Build history of the part. All positions in model axes, mm. A direction names the side the tool comes from. Round coordinates to 2 decimals unless told otherwise and drop trailing zeros. Write each loop counter-clockwise with the first axis right and the second up, starting at its lowest first coordinate (ties: lowest second). Pieces come first, ordered by that corner, then holes.
Item 1: Drop flat-ended pins along their axis: pin 1 Ø3 at (x, z) = (29.5, -20.5) entering from -Y; pin 2 Ø8 at (y, z) = (-28.99, -28.99) entering from +X (3 decimals); pin 3 Ø5 at (x, y) = (15, -27.5) entering from -Z; pin 4 Ø2.5 at (x, y) = (34.5, 27) entering from +Z. Give the stop position or say it passes through.
Item 2: Band-saw the part on A-A, the plane x = 35. Write the cut outline in (y, z).
Item 3: Band-saw the part on C-C, the plane x = 27.5. Write the cut outline in (y, z).
Item 4: Band-saw the part on B-B, the plane x = 6. Write the cut outline in (y, z), then the cut area to 3 significant figures.
Item 5: Wall check: probe 1 along Z at (x, y) = (1.95, 0); probe 2 along Z at (x, y) = (7, 0); probe 3 along Z at (x, y) = (11, -33). Give the ranges that are in metal, low to high.
Item 6: Mould opens along Z. For faces 1 (the flat face through (34, -26, 4)), 2 (the flat face through (31, 0, -26)), 3 (the cylindrical face through (6.577, 49.787, -11.056)) say: +Z half, -Z half, draft (parallel to the pull), parting line (faces both ways), or undercut.
Item 7: 3-axis set-ups, long thin cutter, end or side, ignore diameter. For faces 4 (the conical face through (11.19, 6.17, 11.87)), 5 (the flat face through (22, 21, 21)), 6 (the flat face through (1, 12, 6)), 7 (the flat face through (35, -4, -26)), 8 (the flat face through (34, 26, 4)): which of +Z, -Z, +X, -X, +Y, -Y reach the whole face in a straight line?
Autodesk Inventor part; units mm, degrees
ref_plane "YZ Plane" through (0, 0, 0) normal (1, 0, 0) x (0, 1, 0)
ref_plane "XZ Plane" through (0, 0, 0) normal (0, 1, 0) x (-1, 0, 0)
ref_plane "XY Plane" through (0, 0, 0) normal (0, 0, 1) x (1, 0, 0)
sketch "草图1" plane through (0, 0, 0) normal (0, 1, 0) x (-1, 0, 0)
  line L0 (0, 51) -> (-12, 51)
  line L1 (-12, 51) -> (-12, 29)
  line L2 (-12, 29) -> (-14.5, 29)
  line L3 (-14.5, 29) -> (-14.5, 31)
  line L4 (-14.5, 31) -> (-22, 31)
  line L5 (-22, 31) -> (-22, 29)
  line L6 (-22, 29) -> (-38, 29)
  line L7 (-38, 29) -> (-38, 0)
  line L8 (-38, 0) -> (0, 0)
  line L9 (0, 0) -> (0, 51)
  line L10 (0, 29) -> (-1, 28)
  line L11 (-1, 28) -> (-1, 0)
  line L12 (-38, 25) -> (-15, 22.6998)
  line L13 (-15, 22.6998) -> (-15, 0)
  line L14 (7.6, 0) -> (-45.6, 0)
  dimension "d2" = 51
  dimension "d4" = 26
  dimension "d5" = 12
  dimension "d6" = 31
  dimension "d7" = 29
  dimension "d8" = 10
  dimension "d9" = 2.5
  dimension "d10" = 29
  dimension "d11" = 45
  dimension "d12" = 1
  dimension "d13" = 15
  dimension "d14" = 25
  dimension "d15" = 84.289
revolve "旋转1" add sketch "草图1" angle 360 about axis through (-10, 0, 0) along (1, 0, 0) contours L9 L10 L11 L8 L13 L12 L7 L6 L5 L4 L3 L2 L1 L0
sketch "草图2" plane through (0, 0, 0) normal (0, 1, 0) x (-1, 0, 0)
  line L0 (-22, 29) -> (-38, 29)
  line L1 (-38, 29) -> (-31, 29)
  line L2 (-31, 29) -> (-31, -29)
  line L3 (-31, -29) -> (-38, -29)
  line L4 (-38, -29) -> (-38, 29)
  point P0 (0, 0)
  dimension "d17" = 7
extrude "拉伸1" cut sketch "草图2" along normal mid plane 8
sketch "草图3" plane through (0, 0, 0) normal (0, 0, 1) x (1, 0, 0)
  line L0 (38, 4) -> (38, 29)
  line L1 (22, -29) -> (38, -29)
  line L2 (38, 29) -> (31, 29)
  line L3 (31, 29) -> (31, -29)
  line L4 (31, -29) -> (38, -29)
  line L5 (38, -29) -> (38, 29)
  point P0 (0, 0)
  dimension "d20" = 7
extrude "拉伸2" cut sketch "草图3" along normal mid plane 8
sketch "草图4" plane through (0, 0, 0) normal (-1, 0, 0) x (0, 0, 1)
  circle A0 centre (28.9914, 28.9914) radius 4.5
  circle A1 centre (-28.9914, 28.9914) radius 4.5
  circle A2 centre (-28.9914, -28.9914) radius 4.5
  circle A3 centre (28.9914, -28.9914) radius 4.5
  line L0 (28.9914, 28.9914) -> (0, 0)
  line L1 (0, -71.4) -> (0, 71.4)
  dimension "d23" = 9
  dimension "d24" = 41
  dimension "d27" = 360
  dimension "d42" = 45
extrude "拉伸3" cut sketch "草图4" against normal up to surface (12 mm away)
chamfer "倒角1" distance 1 angle 45 1 edges at (0, 0, -51)
fillet "圆角1" radius 5 1 edges at (15, 0, -22.6998)
sketch "草图5" plane through (0, 0, 0) normal (0, 0, 1) x (1, 0, 0)
  line L0 (0, -29) -> (0, 29)
  line L1 (0, 13) -> (3.7633, 13)
  line L2 (3.7633, 13) -> (4.5, 19)
  line L3 (4.5, 19) -> (10.5, 19)
  line L4 (10.5, 19) -> (11.2367, 13)
  line L5 (11.2367, 13) -> (15, 13)
  line L6 (15, 18.1749) -> (15, -18.1749)
  line L7 (0, 13) -> (0, 0)
  line L8 (0, 0) -> (15, 0)
  line L9 (15, 13) -> (15, 0)
  line L10 (-7.6, 0) -> (45.6, 0)
  point P0 (7.5, 19)
  dimension "d35" = 13
  dimension "d36" = 19
  dimension "d37" = 6
  dimension "d38" = 7
  dimension "d39" = 7
  dimension "d40" = 7.5
revolve "旋转2" cut sketch "草图5" angle 360 about axis through (-10, 0, 0) along (1, 0, 0)
equation "\"d2\" = 0.5 * D2"
equation "\"d4\" = M"
equation "\"d5\" = e"
equation "\"d6\" = 0.5 * D"
equation "\"d7\" = 0.5 * D_d"
equation "\"d8\" = e1"
equation "\"d10\" = 0.5 * D_d"
equation "\"d13\" = b1"
equation "\"d14\" = 0.5 * D4"
equation "\"d17\" = h_b"
equation "\"d18\" = b"
equation "\"d20\" = h_b"
equation "\"d21\" = b"
equation "\"d23\" = d0"
equation "\"d24\" = 0.5 * D0"
equation "\"d29\" = b"
equation "\"d35\" = 0.5 * d1"
equation "\"d36\" = 0.5 * d1_D0"
equation "\"d37\" = d1_b"
equation "\"d3\" = 8"
equation "\"d0\" = 9"
equation "\"D\" = 62"
equation "\"D0\" = 82"
equation "\"D2\" = 102"
equation "\"D_d\" = 58"
equation "\"e\" = 12"
equation "\"e1\" = 10"
equation "\"b\" = 8"
equation "\"h_b\" = 7"
equation "\"M\" = 26"
equation "\"b1\" = 15"
equation "\"d1\" = 26"
equation "\"d1_D0\" = 38"
equation "\"d1_b\" = 6"
properties part number "高速轴承透盖" material "灰口铁"
Results:
1. pin 1: stops at y = -21.91
1. pin 2: passes through
1. pin 3: stops at z = -18.33
1. pin 4: stops at z = 13.34
2. outline: (-28.72, -4) arc R29 ccw to (-4, -28.72) - (-4, -24.37) arc R24.7 cw to (-24.37, -4) - close; (-28.72, 4) - (-24.37, 4) arc R24.7 cw to (-4, 24.37) - (-4, 28.72) arc R29 ccw to start; (4, -28.72) arc R29 ccw to (28.72, -4) - (24.37, -4) arc R24.7 cw to (4, -24.37) - close; (4, 24.37) arc R24.7 cw to (24.37, 4) - (28.72, 4) arc R29 ccw to (4, 28.72) - close
3. outline: circle Ø58 at (0, 0); hole circle Ø47.9 at (0, 0)
4. outline: circle Ø102 at (0, 0); hole circle Ø9 at (-28.99, -28.99); hole circle Ø9 at (-28.99, 28.99); hole circle Ø38 at (0, 0); hole circle Ø9 at (28.99, -28.99); hole circle Ø9 at (28.99, 28.99)
4. area: 6,780 mm2
5. probe 1: z = -51 to -13, 13 to 51
5. probe 2: z = -51 to -19, 19 to 51
5. probe 3: z = -38.88 to -31.04, -26.95 to 26.95, 31.04 to 38.88
6. face 1: undercut
6. face 2: draft
6. face 3: parting line
7. face 4: none
7. face 5: +X
7. face 6: -X
7. face 7: +Z, -Z, +X
7. face 8: +X, +Y, -Y
